Geometry: final body of the model. Coordinates: model frame, mm. A direction names the side the tool comes from. Give positions to 0.01 mm unless a question says otherwise; leave off trailing zeros. Order: outer loops, then holes, each group sorted by start corner. A loop starts at its lowest first (then second) coordinate and runs counter-clockwise, first axis right, second up. Notation, with made-up numbers: M 85,4.5 L 99,4.5 A31 cw 99,41.5 Z; hole C 3.5,38 d11. An arc over 180 degrees is marked long. Use CSV: the item, a comma, the result in double quotes.
```python
from build123d import *
from OCP.BRepFilletAPI import BRepFilletAPI_MakeChamfer

# Parameters (mm, degrees)
SKETCH2_W           = 200
SKETCH2_H           = 100
BOSS_EXTRUDE1_DEPTH = 20
FILLET1_R           = 25
SKETCH3_R           = 8
CUT_EXTRUDE2_DEPTH  = 20
SKETCH4_W           = 10
SKETCH4_H           = 100
BOSS_EXTRUDE3_DEPTH = 80
CHAMFER1_SIZE       = 30
CHAMFER1_SIZE2      = 25
SKETCH5_R           = 11
CUT_EXTRUDE3_DEPTH  = 127
SKETCH8_W           = 30.69541184
SKETCH8_H           = 10
BOSS_EXTRUDE4_DEPTH = 30
CHAMFER2_SIZE       = 31


with BuildPart() as part:
    # Sketch2 → Boss-Extrude1 (new body)
    with BuildSketch(Plane(origin=(0, 0, 0), x_dir=(1, 0, 0), z_dir=(0, 1, 0))):
        Rectangle(SKETCH2_W, SKETCH2_H)
    extrude(amount=BOSS_EXTRUDE1_DEPTH)

    # Fillet1
    fillet1_edges = [part.edges().sort_by_distance(p)[0] for p in [
        (100, 10, 50),
        (-100, 10, 50),
        (-100, 10, -50),
        (100, 10, -50),
    ]]
    fillet(fillet1_edges, radius=FILLET1_R)

    # Sketch3 → Cut-Extrude2 (cut)
    with BuildSketch(Plane(origin=(0, 20, 0), x_dir=(1, 0, 0), z_dir=(0, 1, 0))):
        with Locations(Location((-84, -30, 0), (0, 0, 270))):
            Circle(SKETCH3_R)
        with Locations(Location((84, -30, 0), (0, 0, 270))):
            Circle(SKETCH3_R)
        with Locations(Location((84, 30, 0), (0, 0, 270))):
            Circle(SKETCH3_R)
        with Locations(Location((-84, 30, 0), (0, 0, 270))):
            Circle(SKETCH3_R)
        with Locations(Location((0, -30, 0), (0, 0, 270))):
            Circle(SKETCH3_R)
        with Locations(Location((0, 30, 0), (0, 0, 270))):
            Circle(SKETCH3_R)
    extrude(amount=-CUT_EXTRUDE2_DEPTH, mode=Mode.SUBTRACT)

    # Sketch4 → Boss-Extrude3 (add)
    with BuildSketch(Plane(origin=(0, 0, 0), x_dir=(1, 0, 0), z_dir=(0, 1, 0))):
        with Locations((-40, 0)):
            Rectangle(SKETCH4_W, SKETCH4_H)
        with Locations((40, 0)):
            Rectangle(SKETCH4_W, SKETCH4_H)
    extrude(amount=BOSS_EXTRUDE3_DEPTH)

    # Chamfer1: one chamfer whose edges measure the first distance from different faces: ONE call of the kernel's chamfer builder (chamfer() names one face for all edges)
    chamfer1_edges_1 = [part.edges().sort_by_distance(p)[0] for p in [
        (40, 80, -50),
        (-40, 80, -50),
    ]]
    chamfer1_side_1 = [part.faces().sort_by_distance(p)[0] for p in [
        (-73.3, 10, -50),
    ]]
    chamfer1_edges_2 = [part.edges().sort_by_distance(p)[0] for p in [
        (40, 80, 50),
        (-40, 80, 50),
    ]]
    chamfer1_side_2 = [part.faces().sort_by_distance(p)[0] for p in [
        (0, 1.7, 50),
    ]]
    chamfer1 = BRepFilletAPI_MakeChamfer(part.part.solid().wrapped)
    for e in chamfer1_edges_1:
        chamfer1.Add(CHAMFER1_SIZE, CHAMFER1_SIZE2, e.wrapped, chamfer1_side_1[0].wrapped)  # the first distance lies on this face
    for e in chamfer1_edges_2:
        chamfer1.Add(CHAMFER1_SIZE, CHAMFER1_SIZE2, e.wrapped, chamfer1_side_2[0].wrapped)  # the first distance lies on this face
    add(Compound.cast(chamfer1.Shape()), mode=Mode.REPLACE)

    # Sketch5 → Cut-Extrude3 (cut)
    with BuildSketch(Plane(origin=(45, 0, 0), x_dir=(0, 0, -1), z_dir=(1, 0, 0))):
        with Locations((0, 50)):
            Circle(SKETCH5_R)
    extrude(amount=-CUT_EXTRUDE3_DEPTH, mode=Mode.SUBTRACT)

    # Sketch8 → Boss-Extrude4 (add)
    with BuildSketch(Plane(origin=(0, 20, 0), x_dir=(1, 0, 0), z_dir=(0, 1, 0))):
        with Locations((60.34770592, -20)):
            Rectangle(SKETCH8_W, SKETCH8_H)
        with Locations((60.34770592, 20)):
            Rectangle(SKETCH8_W, SKETCH8_H)
        with Locations((-60.34770592, -20)):
            Rectangle(SKETCH8_W, SKETCH8_H)
        with Locations((-60.34770592, 20)):
            Rectangle(SKETCH8_W, SKETCH8_H)
    extrude(amount=BOSS_EXTRUDE4_DEPTH)

    # Chamfer2
    # the kernel refuses this chamfer: 31 mm, written as the material it takes off along each edge
    with BuildSketch(Plane(origin=(-75.69541184, 50, 64.722172627), x_dir=(0.9996219169112968, 0.027495876610586407, 0), z_dir=(0, 0, -1))) as chamfer2_piece_1_section:
        Polygon((CHAMFER2_SIZE * 0.999621916911, CHAMFER2_SIZE * 0.0274958766106), (-CHAMFER2_SIZE * 0.0274958766106, CHAMFER2_SIZE * 0.999621916911), (0, 0), align=None)
    chamfer2_piece_1 = extrude(amount=169.444345254, mode=Mode.PRIVATE)
    chamfer2_piece_1 = split(chamfer2_piece_1, bisect_by=Plane(origin=(-45, 39.85641553, -20), z_dir=(-1, 0, 0)), keep=Keep.TOP, mode=Mode.PRIVATE)
    chamfer2_piece_1 = split(chamfer2_piece_1, bisect_by=Plane(origin=(-65.469394976, 20, -20), z_dir=(0, 1, 0)), keep=Keep.TOP, mode=Mode.PRIVATE)
    add(chamfer2_piece_1, mode=Mode.SUBTRACT)
    with BuildSketch(Plane(origin=(-75.69541184, 50, -64.722172627), x_dir=(0.9996219169112968, 0.027495876610586407, 0), z_dir=(0, 0, 1))) as chamfer2_piece_2_section:
        Polygon((CHAMFER2_SIZE * 0.999621916911, -CHAMFER2_SIZE * 0.0274958766106), (-CHAMFER2_SIZE * 0.0274958766106, -CHAMFER2_SIZE * 0.999621916911), (0, 0), align=None)
    chamfer2_piece_2 = extrude(amount=169.444345254, mode=Mode.PRIVATE)
    chamfer2_piece_2 = split(chamfer2_piece_2, bisect_by=Plane(origin=(-45, 39.85641553, 20), z_dir=(-1, 0, 0)), keep=Keep.TOP, mode=Mode.PRIVATE)
    chamfer2_piece_2 = split(chamfer2_piece_2, bisect_by=Plane(origin=(-65.469394976, 20, 20), z_dir=(0, 1, 0)), keep=Keep.TOP, mode=Mode.PRIVATE)
    add(chamfer2_piece_2, mode=Mode.SUBTRACT)
    with BuildSketch(Plane(origin=(75.69541184, 50, 64.722172627), x_dir=(0.02749587661058618, -0.9996219169112968, 0), z_dir=(0, 0, -1))) as chamfer2_piece_3_section:
        Polygon((CHAMFER2_SIZE * 0.999621916911, CHAMFER2_SIZE * 0.0274958766106), (-CHAMFER2_SIZE * 0.0274958766106, CHAMFER2_SIZE * 0.999621916911), (0, 0), align=None)
    chamfer2_piece_3 = extrude(amount=169.444345254, mode=Mode.PRIVATE)
    chamfer2_piece_3 = split(chamfer2_piece_3, bisect_by=Plane(origin=(65.469394976, 20, -20), z_dir=(0, 1, 0)), keep=Keep.TOP, mode=Mode.PRIVATE)
    chamfer2_piece_3 = split(chamfer2_piece_3, bisect_by=Plane(origin=(45, 39.85641553, -20), z_dir=(1, 0, 0)), keep=Keep.TOP, mode=Mode.PRIVATE)
    add(chamfer2_piece_3, mode=Mode.SUBTRACT)
    with BuildSketch(Plane(origin=(75.69541184, 50, 104.722172627), x_dir=(0.02749587661058618, -0.9996219169112968, 0), z_dir=(0, 0, -1))) as chamfer2_piece_4_section:
        Polygon((CHAMFER2_SIZE * 0.999621916911, CHAMFER2_SIZE * 0.0274958766106), (-CHAMFER2_SIZE * 0.0274958766106, CHAMFER2_SIZE * 0.999621916911), (0, 0), align=None)
    chamfer2_piece_4 = extrude(amount=169.444345254, mode=Mode.PRIVATE)
    chamfer2_piece_4 = split(chamfer2_piece_4, bisect_by=Plane(origin=(65.469394976, 20, 20), z_dir=(0, 1, 0)), keep=Keep.TOP, mode=Mode.PRIVATE)
    chamfer2_piece_4 = split(chamfer2_piece_4, bisect_by=Plane(origin=(45, 39.85641553, 20), z_dir=(1, 0, 0)), keep=Keep.TOP, mode=Mode.PRIVATE)
    add(chamfer2_piece_4, mode=Mode.SUBTRACT)


solid = part.part
```
1. Section D-D, the plane x = -84. Return the cut outline in (y, z), plus the area to 3 significant figures.
Answer:
outline,"M 0,-48.32 L 20,-48.32 L 20,-38 L 0,-38 Z; M 0,-22 L 20,-22 L 20,22 L 0,22 Z; M 0,38 L 20,38 L 20,48.32 L 0,48.32 Z"
area,"1,290 mm2"
2. Line query: line 1 (X direction, y = 68.5, z = -31); line 2 (Z direction, x = 40.25, y = 50); line 3 (Y direction, x = -12.5, z = -39). Output: solid intervals per line, ascending.
Answer:
line 1,"-45 to -35, 35 to 45"
line 2,"-50 to -11, 11 to 50"
line 3,"0 to 20"
3. Reachability of faces 1 (the face through (-53, 28, -15)), 2 (the face through (56, 31, 25)), 3 (the face through (56, 31, 15)) from +Z, -Z, +X, -X, +Y, -Y: full face, straight path, thin tool, end or side. Return the list, or none.
Answer:
face 1,"-X, +Y"
face 2,"+Z, +X, +Y"
face 3,"+X, +Y"
4. Section B-B, the plane z = 0. Return the cut outline in (x, y), plus the area to 3 significant figures.
Answer:
outline,"M -100,0 L 100,0 L 100,20 L 45,20 L 45,39 L 35,39 L 35,20 L -35,20 L -35,39 L -45,39 L -45,20 L -100,20 Z; M -45,61 L -35,61 L -35,80 L -45,80 Z; M 35,61 L 45,61 L 45,80 L 35,80 Z"
area,"4,760 mm2"
5. Section A-A, the plane x = -42. Return the cut outline in (y, z).
Answer:
outline,"M 0,-50 L 50,-50 L 80,-25 L 80,25 L 50,50 L 0,50 Z; hole C 50,0 d22"
6. Pin query (flat end, axial travel): pin 1 Ø18 at (y, z) = (49, -16.5) entering from +X; pin 2 Ø21 at (x, z) = (-7, -19.5) entering from +Y; pin 3 Ø4 at (x, z) = (1.5, -24.5) entering from +Y (3 decimals); pin 4 Ø5 at (y, z) = (12, 33.5) entering from -X. Return the tip coordinate at first contact, or that it passes through.
Answer:
pin 1,"x = 54.7"
pin 2,"y = 20"
pin 3,"through"
pin 4,"x = -99.27"
7. Section C-C, the plane y = 59. Return the cut outline in (x, z), plus the area to 3 significant figures.
Answer:
outline,"M -45,-42.5 L -35,-42.5 L -35,-6.32 L -45,-6.32 Z; M -45,6.32 L -35,6.32 L -35,42.5 L -45,42.5 Z; M 35,-42.5 L 45,-42.5 L 45,-6.32 L 35,-6.32 Z; M 35,6.32 L 45,6.32 L 45,42.5 L 35,42.5 Z"
area,"1,450 mm2"
8. Pull-direction query (Y, two-part tool) for faces 4 (the face through (40.07, 57.43, 8.11)), 5 (the face through (-53, 28, 15)), 6 (the face through (60.056, 34.64, -19.93)); classes: +Y half, -Y half, draft (parallel to the pull), parting line (faces both ways), or undercut.
Answer:
face 4,"undercut"
face 5,"draft"
face 6,"+Y half"
